```python
from build123d import *

# Parameters (mm, degrees)
F0_R     = 3
F1_DEPTH = 2


with BuildPart() as f1:
    # F0 (on Top) → F1 (new body)
    with BuildSketch(Plane.XY):
        with BuildLine():
            Line((0, -12.255436), (-1.6, -12.255436))
            Line((-1.6, -12.255436), (-1.6, -15.58141))
            ThreePointArc((-1.6, -15.58141), (-3.805204, -16.750233), (-4.974027, -18.955436))
            Line((-4.974027, -18.955436), (-8.3, -18.955436))
            Line((-8.3, -18.955436), (-8.3, -20.555436))
            Line((-8.3, -20.555436), (-4.974027, -20.555436))
            ThreePointArc((-4.974027, -20.555436), (-3.805204, -22.76064), (-1.6, -23.929463))
            Line((-1.6, -23.929463), (-1.6, -27.255436))
            Line((-1.6, -27.255436), (0, -27.255436))
            Line((0, -27.255436), (0, -23.929463))
            ThreePointArc((0, -23.929463), (2.205204, -22.76064), (3.374027, -20.555436))
            Line((3.374027, -20.555436), (6.7, -20.555436))
            Line((6.7, -20.555436), (6.7, -18.955436))
            Line((6.7, -18.955436), (3.374027, -18.955436))
            ThreePointArc((3.374027, -18.955436), (2.205204, -16.750233), (0, -15.58141))
            Line((0, -15.58141), (0, -12.255436))
        make_face()
        with Locations((-0.8, -19.755436)):
            Circle(F0_R, mode=Mode.SUBTRACT)
    extrude(amount=F1_DEPTH)


solid = f1.part
```
Could you check a few things on this model? Use its own coordinates, in mm. A direction names the side the tool comes from. Give positions to 0.01 mm unless a question says otherwise; leave off trailing zeros. Order: outer loops, then holes, each group sorted by start corner. A loop starts at its lowest first (then second) coordinate and runs counter-clockwise, first axis right, second up.
Q1. I'm going to push flat-ended pins straight in: P1, Ø1, axis at x = -6.5, z = 1, coming from the +Y side; P2, Ø1, axis at y = -14, z = 1.5, coming from the -X side; P3, Ø0.6, axis at x = -7, z = 1, coming from the -Y side. Where does each tip first touch, or does it pass through?
Q2. If I drill on line 1 along Y through (x, z) = (-0.8, 1.5); line 2 along Y through (x, z) = (-7.5, 0.9); line 3 along X through (y, z) = (-13.75, 1), over which ranges is the centre line in solid material (lowest first)?
Q3. Suppose I cut it at B-B, the plane z = 0.6. Write out the boundary of the cut face in (x, y).
Q4. Suppose I cut it at C-C, the plane x = 1.75. Write out the boundary of the cut face in (y, z), and give its area (3 significant figures).
Q5. Suppose I cut it at A-A, the plane x = -0.8. Write out the boundary of the cut face in (y, z).
Q6. Suppose I cut it at D-D, the plane y = -25.5. Write out the boundary of the cut face in (x, z).
Q7. For faces 1 (the flat face through (-7, -20.555, 1)), 2 (the flat face through (0, -14, 1)), 3 (the flat face through (-1.6, -14, 1)), which set-ups out of +Z, -Z, +X, -X, +Y, -Y let a thin tool reach every point of the face, with its end or its side?
Solution:
1. P1: stops at y = -18.96
1. P2: stops at x = -1.6
1. P3: stops at y = -20.56
2. line 1: y = -27.26 to -22.76, -16.76 to -12.26
2. line 2: y = -20.56 to -18.96
2. line 3: x = -1.6 to 0
3. outline: (-8.3, -20.56) - (-4.97, -20.56) arc R4.25 ccw to (-1.6, -23.93) - (-1.6, -27.26) - (0, -27.26) - (0, -23.93) arc R4.25 ccw to (3.37, -20.56) - (6.7, -20.56) - (6.7, -18.96) - (3.37, -18.96) arc R4.25 ccw to (0, -15.58) - (0, -12.26) - (-1.6, -12.26) - (-1.6, -15.58) arc R4.25 ccw to (-4.97, -18.96) - (-8.3, -18.96) - close; hole circle Ø6 at (-0.8, -19.76)
4. outline: (-23.16, 0) - (-21.34, 0) - (-21.34, 2) - (-23.16, 2) - close; (-18.18, 0) - (-16.36, 0) - (-16.36, 2) - (-18.18, 2) - close
4. area: 7.28 mm2
5. outline: (-27.26, 0) - (-22.76, 0) - (-22.76, 2) - (-27.26, 2) - close; (-16.76, 0) - (-12.26, 0) - (-12.26, 2) - (-16.76, 2) - close
6. outline: (-1.6, 0) - (0, 0) - (0, 2) - (-1.6, 2) - close
7. face 1: +Z, -Z, -X, -Y
7. face 2: +Z, -Z, +X, +Y
7. face 3: +Z, -Z, -X, +Y
